Could you check a few things on this drawing? It's one solid part, dimensions in mm from its lowest x, y, z. Give positions to 0.01 mm unless a question says otherwise; leave off trailing zeros. Write each loop counter-clockwise with the first axis right and the second up, starting at its lowest first coordinate (ties: lowest second). Pieces come first, ordered by that corner, then holes. Notation, with made-up numbers: M 0,18 L 29,18 A29 ccw 29,51 Z; hole C 67.5,88.5 d10. An arc over 180 degrees is marked long. Write each question's results on one line, items separated by ' | '.
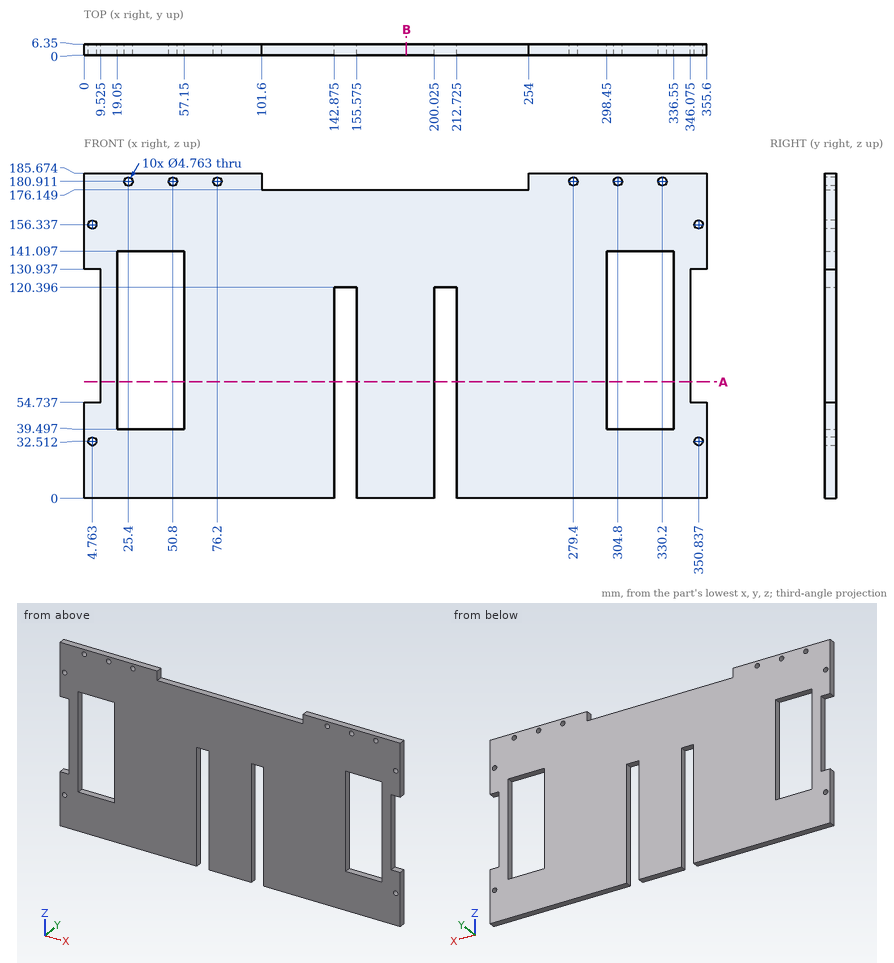
Item 1: If I drill on line 1 (X direction, y = 3, z = 139.5); line 2 (X direction, y = 2.25, z = 21) (1 decimal); line 3 (Z direction, x = 304.8, y = 1.75) (1 decimal), over which ranges is the centre line in solid material (lowest first)? Write a range as from..to.
Geometry says:
line 1: x = 0..19.05, 57.15..298.45, 336.55..355.6 | line 2: x = 0..142.9, 155.6..200, 212.7..355.6 | line 3: z = 0..39.5, 141.1..178.5, 183.3..185.7
Item 2: I want a section at B-B, the plane x = 184. Please give me the cut outline in (y, z).
Geometry says:
outline: M 0,0 L 6.35,0 L 6.35,176.15 L 0,176.15 Z
Item 3: I want a section at A-A, the plane z = 66.5. Give the number of separate pieces and of enclosed holes in the cut face, and give its area (3 significant figures).
Geometry says:
separate pieces: 5 | enclosed holes: 0 | area: 1,490 mm2
Item 4: I'm going to push flat-ended pins straight in: pin 1 (6 mm diameter, centred on x = 330.2, z = 180.91, fed in from +Y); pin 2 (3 mm diameter, centred on x = 140.5, y = 4.5, fed in from +Z); pin 3 (3 mm diameter, centred on x = 304.8, z = 180.91, fed in from +Y); pin 4 (3 mm diameter, centred on x = 205.5, y = 4, fed in from -Z). Where does each tip first touch, or does it pass through?
Geometry says:
pin 1: stops at y = 6.35 | pin 2: stops at z = 176.15 | pin 3: passes through | pin 4: stops at z = 120.4
